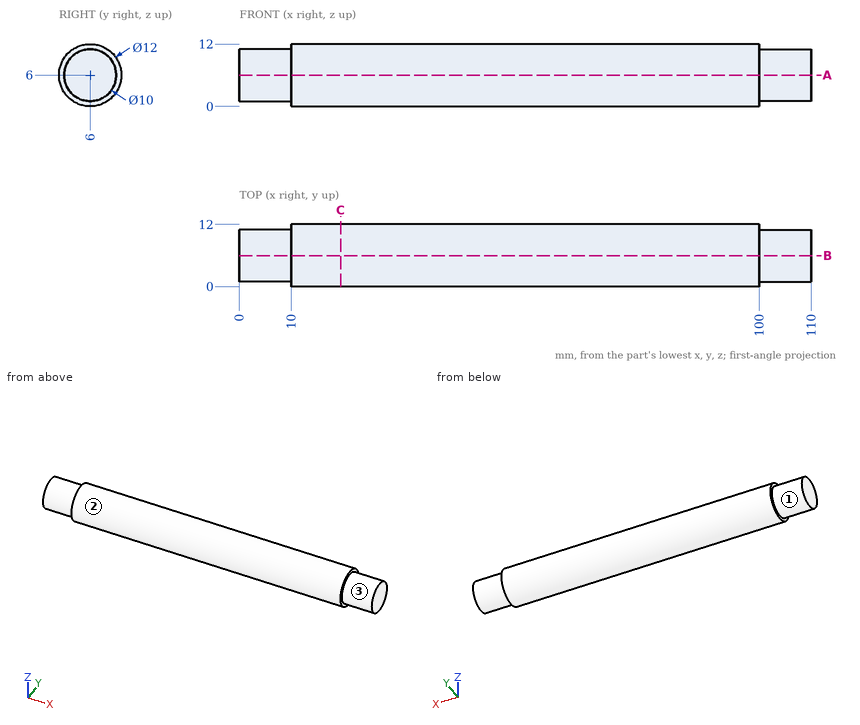
Could you check a few things on this drawing? It's one solid part, dimensions in mm from its lowest x, y, z. A direction names the side the tool comes from. Give positions to 0.01 mm unless a question says otherwise; leave off trailing zeros. Order: outer loops, then holes, each group sorted by start corner. A loop starts at its lowest first (then second) coordinate and runs counter-clockwise, first axis right, second up. Notation, with made-up numbers: (85.25, 54) - (113.25, 54) arc R25 cw to (113.25, 80) - close; hole circle Ø3 at (-35.5, 34). An arc over 180 degrees is marked (long way). One line per question, with ' | ' between items. Start each with the question number.
Item 1: For the marked faces 1, 2 and 3, which set-ups out of +Z, -Z, +X, -X, +Y, -Y let a thin tool reach every point of the face, with its end or its side?
Item 2: I want a section at C-C on x = 19.5. Write out the boundary of the cut face in (y, z), then the cut area to 3 significant figures.
Item 3: I'm going to push flat-ended pins straight in: pin 1 Ø1 at (x, y) = (94.5, 2.5) entering from +Z; pin 2 Ø1.5 at (x, y) = (35, 1.5) entering from +Z; pin 3 Ø4 at (x, y) = (14, 3) entering from +Z. Where does each tip first touch, or does it pass through?
Item 4: I need wall thicknesses on probe 1 along Y at (x, z) = (21, 5.75); probe 2 along X at (y, z) = (2, 10); probe 3 along Z at (x, y) = (25, 2.5). Which ranges of each line are inside material? Lowest first, please. Write a range as [from, to].
Item 5: I want a section at A-A on z = 6. Write out the boundary of the cut face in (x, y), then the cut area to 3 significant figures.
Verdict:
1) face 1: -X | face 2: +X, -X | face 3: +X
2) outline: circle Ø12 at (6, 6) | area: 113 mm^2
3) pin 1: z = 11.2 | pin 2: z = 10.68 | pin 3: z = 11.92
4) probe 1: [0.01, 11.99] | probe 2: [10, 100] | probe 3: [1.13, 10.87]
5) outline: (0, 1) - (10, 1) - (10, 0) - (100, 0) - (100, 1) - (110, 1) - (110, 11) - (100, 11) - (100, 12) - (10, 12) - (10, 11) - (0, 11) - close | area: 1,280 mm^2
